Study the drawing (mm; zero at the part's minimum x, y, z) and answer. Round coordinates to 2 decimals unless told otherwise and drop trailing zeros. Write each loop counter-clockwise with the first axis right and the second up, starting at its lowest first coordinate (ties: lowest second). Pieces come first, ordered by that corner, then holes.
(1) A cutting plane is placed at B-B, the plane y = 120. Give the vertices of the cut face in (x, z), and give its area (3 significant figures).
(2) The mould has two halves that part along Z. Classify the marked faces 1 and 2: +Z half, -Z half, draft (parallel to the pull), parting line (faces both ways), or undercut.
(3) A cutting plane is placed at C-C, the plane z = 1.55. Give the vertices of the cut face in (x, y), and give its area (3 significant figures).
(4) A cutting plane is placed at A-A, the plane x = 106. Give the vertices of the cut face in (y, z), and give its area (3 significant figures).
(5) Each of these flat-tipped pins is pushed along its axis until it touches: pin 1 Ø1 at (x, z) = (137, 2.5) entering from +Y; pin 2 Ø0.9 at (x, z) = (91.5, 1.5) entering from -Y. Where does it stop, or does it pass through?
(6) A cutting plane is placed at D-D, the plane x = 153. Give the vertices of the cut face in (y, z).
(7) Find the intervals of material crossed by probe 1 along Y at (x, z) = (153, 1.3); probe 2 along Y at (x, z) = (65.5, 1.7); probe 3 along X at (y, z) = (18.5, 0.25), in increasing order.
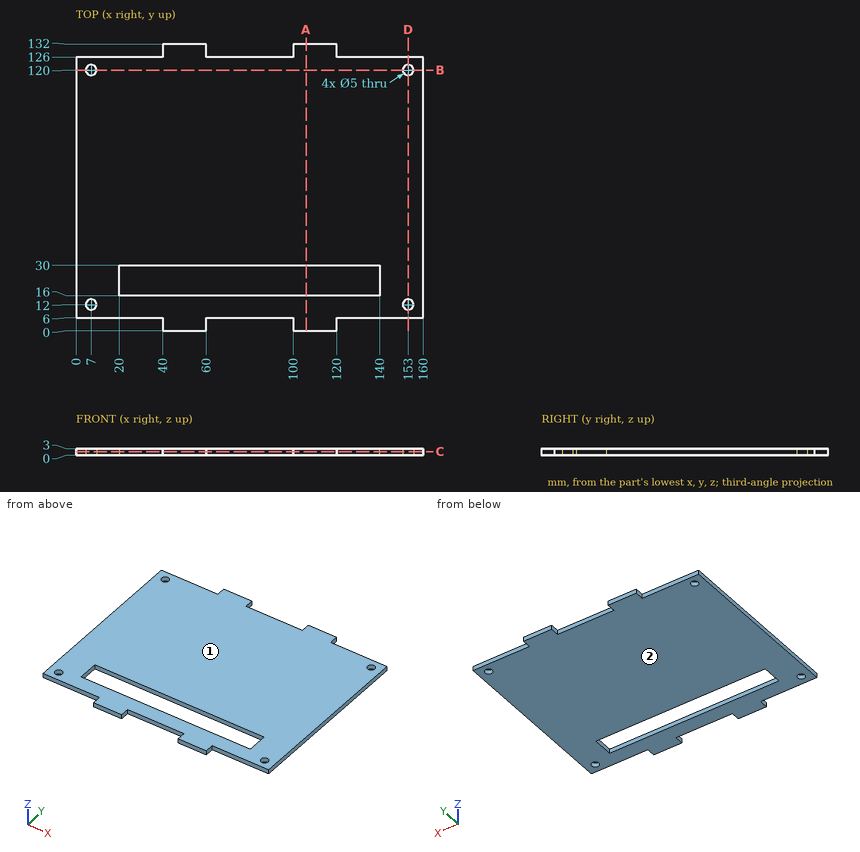
Solutions:
1. outline: (0, 0) - (4.5, 0) - (4.5, 3) - (0, 3) - close; (9.5, 0) - (150.5, 0) - (150.5, 3) - (9.5, 3) - close; (155.5, 0) - (160, 0) - (160, 3) - (155.5, 3) - close
1. area: 450 mm2
2. face 1: +Z half
2. face 2: -Z half
3. outline: (0, 6) - (40, 6) - (40, 0) - (60, 0) - (60, 6) - (100, 6) - (100, 0) - (120, 0) - (120, 6) - (160, 6) - (160, 126) - (120, 126) - (120, 132) - (100, 132) - (100, 126) - (60, 126) - (60, 132) - (40, 132) - (40, 126) - (0, 126) - close; hole circle Ø5 at (7, 12); hole circle Ø5 at (7, 120); hole (20, 16) - (140, 16) - (140, 30) - (20, 30) - close; hole circle Ø5 at (153, 12); hole circle Ø5 at (153, 120)
3. area: 17,900 mm2
4. outline: (0, 0) - (16, 0) - (16, 3) - (0, 3) - close; (30, 0) - (132, 0) - (132, 3) - (30, 3) - close
4. area: 354 mm2
5. pin 1: stops at y = 126
5. pin 2: stops at y = 6
6. outline: (6, 0) - (9.5, 0) - (9.5, 3) - (6, 3) - close; (14.5, 0) - (117.5, 0) - (117.5, 3) - (14.5, 3) - close; (122.5, 0) - (126, 0) - (126, 3) - (122.5, 3) - close
7. probe 1: y = 6 to 9.5, 14.5 to 117.5, 122.5 to 126
7. probe 2: y = 6 to 16, 30 to 126
7. probe 3: x = 0 to 20, 140 to 160
